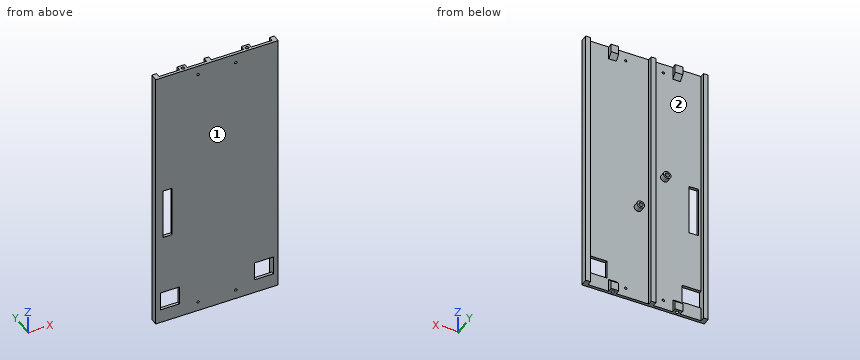
Autodesk Inventor part; units mm, degrees
ref_plane "YZ Plane" through (0, 0, 0) normal (1, 0, 0) x (0, 1, 0)
ref_plane "XZ Plane" through (0, 0, 0) normal (0, 1, 0) x (-1, 0, 0)
ref_plane "XY Plane" through (0, 0, 0) normal (0, 0, 1) x (1, 0, 0)
sketch "Sketch1" plane through (0, 0, 0) normal (0, 1, 0) x (-1, 0, 0)
  line L0 (65, -145) -> (-65, -145)
  line L1 (-65, -145) -> (-65, 145)
  line L2 (-65, 145) -> (65, 145)
  line L3 (65, 145) -> (65, -145)
  line L4 (65, 0) -> (-65, 0) construction
  line L5 (0, -145) -> (0, 145) construction
  point P0 (0, 0)
  point P1 (0, 0)
  dimension "d0" = 130
  dimension "d1" = 290
extrude "Extrusion1" add sketch "Sketch1" along normal blind 3
sketch "Sketch2" plane through (0, 0, 0) normal (0, -1, 0) x (1, 0, 0)
  line L0 (65, -145) -> (-65, -145) construction
  line L1 (0, -145) -> (0, 145) construction
  line L2 (-65, 145) -> (65, 145) construction
  line L3 (65, 145) -> (65, -145) construction
  line L4 (65, 0) -> (-65, 0) construction
  line L5 (-65, -145) -> (-65, 145) construction
  line L6 (-38, -145) -> (-30, -145)
  line L7 (-30, -145) -> (-30, -131)
  line L8 (-30, -131) -> (-38, -131)
  line L9 (-38, -131) -> (-38, -145)
  line L10 (38, -145) -> (30, -145)
  line L11 (30, -145) -> (30, -131)
  line L12 (30, -131) -> (38, -131)
  line L13 (38, -131) -> (38, -145)
  line L14 (-38, 145) -> (-30, 145)
  line L15 (-30, 145) -> (-30, 131)
  line L16 (-30, 131) -> (-38, 131)
  line L17 (-38, 131) -> (-38, 145)
  line L18 (30, 145) -> (30, 131)
  line L19 (38, 131) -> (38, 145)
  line L20 (30, 131) -> (38, 131)
  line L21 (38, 145) -> (30, 145)
  point P0 (0, 0)
  dimension "d4" = 8
  dimension "d5" = 14
  dimension "d6" = 30
extrude "Extrusion2" add sketch "Sketch2" against normal blind 8
chamfer "Chamfer1" distance 5 angle 45 4 edges at (-34, 8, 131) (34, 8, 131) (-34, 8, -131) (34, 8, -131)
sketch "Sketch3" plane through (65, 0, -145) normal (0, 0, -1) x (-1, 0, 0)
  line L0 (65, 0) -> (65, 3) construction
  line L1 (35, 3) -> (95, 3) construction
  circle A0 centre (31, 4) radius 1.75
  line L2 (27, 8) -> (35, 8)
  line L3 (35, 3) -> (35, 8)
  circle A1 centre (99, 4) radius 1.75
  dimension "d12" = 3.5
  dimension "d13" = 4
  dimension "d14" = 4
extrude "Extrusion3" cut sketch "Sketch3" against normal blind 6
sketch "Sketch4" plane through (-65, 0, 145) normal (0, 0, 1) x (1, 0, 0)
  circle A0 centre (99, 4) radius 1.75
  circle A1 centre (31, 4) radius 1.75
  point P0 (65, 0)
extrude "Extrusion4" cut sketch "Sketch4" against normal blind 6
sketch "Sketch5" plane through (0, 3, 0) normal (0, 1, 0) x (1, 0, 0)
  line L0 (-60, 130) -> (-40, 130)
  line L1 (-40, 130) -> (-40, 110)
  line L2 (-40, 110) -> (-60, 110)
  line L3 (-60, 110) -> (-60, 130)
  line L4 (-38, 145) -> (-65, 145)
  line L5 (-65, 145) -> (-65, -145)
  line L6 (-65, 145) -> (65, 145) construction
  line L7 (0, 145) -> (0, -145) construction
  line L8 (-30, -145) -> (30, -145) construction
  line L9 (60, 130) -> (40, 130)
  line L10 (40, 130) -> (40, 110)
  line L11 (40, 110) -> (60, 110)
  line L12 (60, 110) -> (60, 130)
  point P0 (0, 0)
  dimension "d19" = 20
  dimension "d20" = 20
  dimension "d21" = 15
  dimension "d22" = 5
extrude "Extrusion5" cut sketch "Sketch5" against normal up to next
sketch "Sketch7" plane through (0, 3, 0) normal (0, 1, 0) x (1, 0, 0)
  line L0 (44, -14) -> (-25, -14) construction
  line L1 (-25, -14) -> (-25, 70) construction
  line L2 (-25, 70) -> (44, 70) construction
  line L3 (44, 70) -> (44, -14) construction
  line L4 (9.5, -14) -> (9.5, 70) construction
  line L5 (44, 28) -> (-25, 28) construction
  line L6 (-65, 145) -> (-65, -145) construction
  circle A0 centre (-21, -10) radius 4
  circle A1 centre (-21, -10) radius 2.25
  circle A2 centre (7, 35) radius 4
  circle A3 centre (7, 35) radius 2.25
  point P0 (0, 0)
  point P1 (40, 110)
  dimension "d39" = 69
  dimension "d40" = 84
  dimension "d41" = 40
  dimension "d42" = 40
  dimension "d43" = 8
  dimension "d44" = 4
  dimension "d45" = 4
  dimension "d46" = 4.5
  dimension "d49" = 8
  dimension "d50" = 49
  dimension "d51" = 32
  dimension "d52" = 4.5
extrude "Extrusion7" add sketch "Sketch7" along normal blind 6
sketch "Sketch8" plane through (0, 3, 0) normal (0, 1, 0) x (1, 0, 0)
  line L0 (-57.5, 45) -> (-47.5, 45)
  line L1 (-47.5, 45) -> (-47.5, -10)
  line L2 (-47.5, -10) -> (-57.5, -10)
  line L3 (-57.5, -10) -> (-57.5, 45)
  line L4 (-38, 145) -> (-65, 145)
  line L5 (-65, 145) -> (-65, -145)
  point P0 (0, 0)
  dimension "d53" = 10
  dimension "d54" = 100
  dimension "d55" = 55
  dimension "d56" = 7.5
extrude "Extrusion8" cut sketch "Sketch8" against normal blind 6
sketch "Sketch9" plane through (0, 3, 0) normal (0, 1, 0) x (1, 0, 0)
  line L0 (65, -145) -> (-65, -145) construction
  line L1 (0, -145) -> (0, 145) construction
  line L2 (-65, 145) -> (65, 145) construction
  line L3 (65, 145) -> (65, -145) construction
  line L4 (65, 0) -> (-65, 0) construction
  line L5 (-65, -145) -> (-65, 145) construction
  line L6 (30, 145) -> (30, 131) construction
  line L7 (30, 135) -> (-30, 135) construction
  line L8 (-30, 131) -> (-30, 145) construction
  circle A0 centre (20, 135) radius 1.25
  circle A1 centre (-20, 135) radius 1.25
  circle A2 centre (20, -135) radius 1.25
  circle A3 centre (-20, -135) radius 1.25
  point P0 (0, 0)
  point P1 (30, 136)
  point P2 (-30, 136)
  dimension "d60" = 10
  dimension "d61" = 2.5
  dimension "d62" = 40
extrude "Extrusion9" cut sketch "Sketch9" against normal blind 10
sketch "Sketch10" plane through (0, 3, 0) normal (0, 1, 0) x (1, 0, 0)
  line L0 (65, -145) -> (-65, -145) construction
  line L1 (0, -145) -> (0, 145) construction
  line L2 (-65, 145) -> (65, 145) construction
  line L3 (-65, -145) -> (-65, 145)
  line L4 (-65, -145) -> (-60, -145)
  line L5 (-60, -145) -> (-60, 145)
  line L6 (-60, 145) -> (-65, 145)
  line L7 (-65, 145) -> (-65, -145)
  line L8 (65, -145) -> (65, 145)
  line L9 (65, -145) -> (60, -145)
  line L10 (60, -145) -> (60, 145)
  line L11 (60, 145) -> (65, 145)
  line L12 (65, 145) -> (65, -145)
  point P0 (0, 0)
  dimension "d65" = 5
extrude "Extrusion10" add sketch "Sketch10" along normal blind 5
sketch "Sketch11" plane through (0, 3, 0) normal (0, 1, 0) x (1, 0, 0)
  line L0 (65, -145) -> (-65, -145)
  line L1 (-65, 145) -> (65, 145)
  line L2 (-4.5, -145) -> (-9.5, -145)
  line L3 (-9.5, -145) -> (-9.5, 145)
  line L4 (-9.5, 145) -> (-4.5, 145)
  line L5 (-4.5, 145) -> (-4.5, -145)
  circle A0 centre (-21, -10) radius 4
  point P0 (0, 0)
  dimension "d68" = 5
  dimension "d69" = 11.5
extrude "Extrusion11" add sketch "Sketch11" along normal blind 5 contours L0 L3 L1 L5
properties part number "electronics_board_tray"
Can you work these out from the model? Positions are in its coordinate system, mm. Face numbers are marked on the shaded views. Coordinates: 2 decimals unless noted, no trailing zeros. Write each loop counter-clockwise with the first axis right and the second up, starting at its lowest first coordinate (ties: lowest second). Pieces come first, ordered by that corner, then holes. Notation, with made-up numbers: (-16, 88.25) -> (36, 88.25) arc R12 ccw to (36, 99.25) -> close; hole circle Ø7 at (-37.75, 12). An arc over 180 degrees is marked (long way). Write each question's results on one line, items separated by ' | '. Start each with the question number.
Item 1: If we section it at D-D, the plane x = 15: Write out the boundary of the cut face in (y, z).
Item 2: Please list where these lines run through material, in increasing order: probe 1 along X at (y, z) = (2.75, -122.5); probe 2 along X at (y, z) = (5, 10); probe 3 along X at (y, z) = (6.5, 33.5).
Item 3: Thinking about a two-plate mould opening in X: for the marked faces 1 and 2, which applies, released by +X, released by -X, zero draft, split by the parting line, or undercut?
Item 4: If we section it at A-A, the plane z = -25.5: Write out the boundary of the cut face in (x, y), and give its area (3 significant figures).
Item 5: I'm going to push flat-ended pins straight in: P1, Ø2.5, axis at x = 63, z = 7, coming from the +Y side; P2, Ø1.5, axis at x = -48.5, z = 66, coming from the +Y side. Where does each tip first touch, or does it pass through?
Item 6: If we section it at B-B, the plane z = -126.5: Write out the boundary of the cut face in (x, y).
Item 7: If we section it at C-C, the plane z = 57.5: Write out the boundary of the cut face in (x, y).
Answer block:
1) outline: (0, -145) -> (3, -145) -> (3, 145) -> (0, 145) -> close
2) probe 1: -65 to -60, -40 to 40, 60 to 65 | probe 2: -65 to -60, -25 to -23.25, -18.75 to -17, -9.5 to -4.5, 60 to 65 | probe 3: -65 to -60, -9.5 to -4.5, 60 to 65
3) face 1: zero draft | face 2: undercut
4) outline: (-65, 0) -> (-57.5, 0) -> (-57.5, 3) -> (-60, 3) -> (-60, 8) -> (-65, 8) -> close; (-47.5, 0) -> (65, 0) -> (65, 8) -> (60, 8) -> (60, 3) -> (-4.5, 3) -> (-4.5, 8) -> (-9.5, 8) -> (-9.5, 3) -> (-47.5, 3) -> close | area: 435 mm²
5) P1: y = 8 | P2: y = 3
6) outline: (-65, 0) -> (-60, 0) -> (-60, 8) -> (-65, 8) -> close; (-40, 0) -> (40, 0) -> (40, 3) -> (-4.5, 3) -> (-4.5, 8) -> (-9.5, 8) -> (-9.5, 3) -> (-40, 3) -> close; (60, 0) -> (65, 0) -> (65, 8) -> (60, 8) -> close
7) outline: (-65, 0) -> (65, 0) -> (65, 8) -> (60, 8) -> (60, 3) -> (-4.5, 3) -> (-4.5, 8) -> (-9.5, 8) -> (-9.5, 3) -> (-60, 3) -> (-60, 8) -> (-65, 8) -> close
